For this review, use the dimensioned drawing (mm, ordinates from the lowest corner) and the shaded views. A direction names the side the tool comes from. Give positions to 0.01 mm unless a question says otherwise; leave off trailing zeros. Order: outer loops, then holes, each group sorted by start corner. A loop starts at its lowest first (then second) coordinate and runs counter-clockwise, first axis right, second up. Notation, with made-up numbers: (38, -10.5) -> (62, -10.5) arc R31 ccw to (62, 28.5) -> close; hole circle Ø3 at (81, -11.75). An arc over 180 degrees is marked (long way). One line per item, written item: value. Start each with the question number.
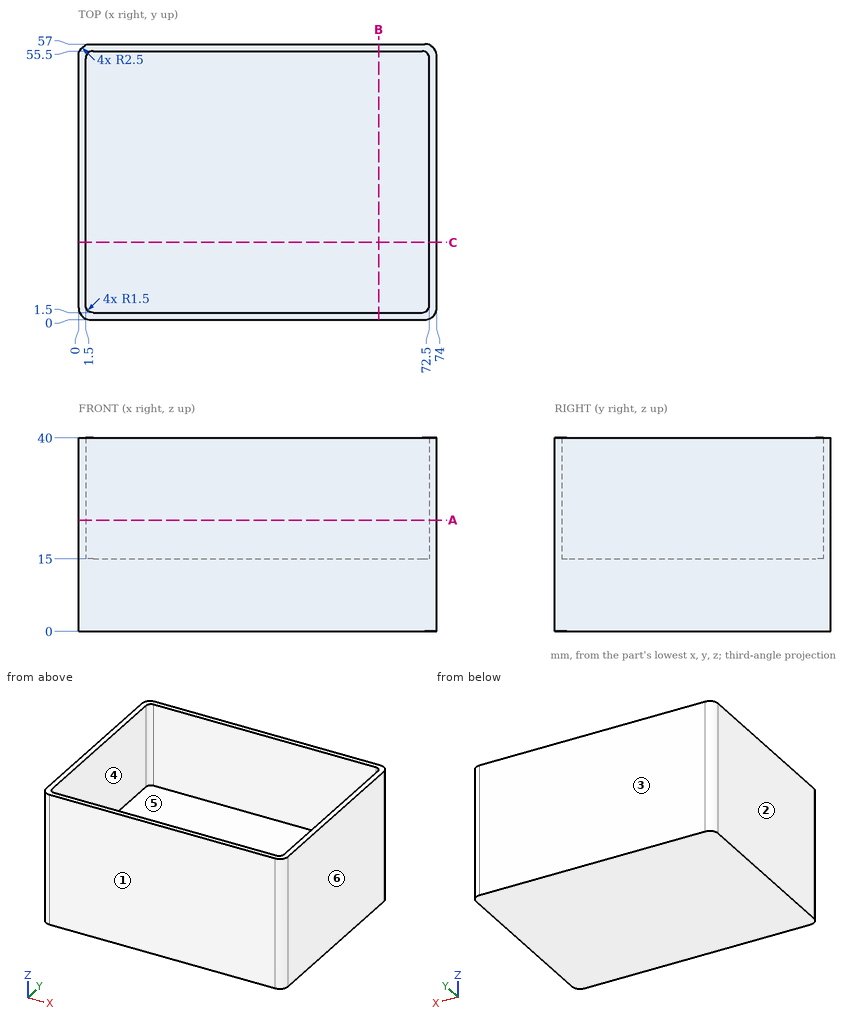
Q1. Take a section at C-C (y = 16). State the section outline as (x, z) points.
Q2. For pin 1 Ø10 at (x, y) = (33.5, 39.5) entering from +Z; pin 2 Ø6 at (x, z) = (56.5, 10) entering from -Y, all flat-tipped, find the tip position at first contact; note any pin that passes through.
Q3. For line 1 along Y through (x, z) = (28, 22); line 2 along X through (y, z) = (28, 29); line 3 along Z through (x, y) = (23, 6), list the stretches that pass through material, from the lowest coordinate up.
Q4. For the marked faces 5 and 6, list the 3-axis set-ups (+Z, -Z, +X, -X, +Y, -Y) from which the entire face can be reached by the end or side of a thin tool; tool diameter is ignored.
Q5. Take a section at B-B (x = 62). State the section outline as (y, z) points, and give its area (3 significant figures).
Q6. Take a section at A-A (z = 23). State the section outline as (x, y) points, and give its area (3 significant figures).
Q7. Mouldability with a two-part tool opening along Y and no side actions: class the marked faces 1, 2, 3 and 4 as pulls with the +Y half, pulls with the -Y half, needs draft (parallel to the pull), parting line crosses it, or undercut.
Answers below:
1. outline: (0, 0) -> (74, 0) -> (74, 40) -> (72.5, 40) -> (72.5, 15) -> (1.5, 15) -> (1.5, 40) -> (0, 40) -> close
2. pin 1: stops at z = 15
2. pin 2: stops at y = 0
3. line 1: y = 0 to 1.5, 55.5 to 57
3. line 2: x = 0 to 1.5, 72.5 to 74
3. line 3: z = 0 to 15
4. face 5: +Z
4. face 6: +Z, -Z, +X, +Y, -Y
5. outline: (0, 0) -> (57, 0) -> (57, 40) -> (55.5, 40) -> (55.5, 15) -> (1.5, 15) -> (1.5, 40) -> (0, 40) -> close
5. area: 930 mm²
6. outline: (0, 2.5) arc R2.5 ccw to (2.5, 0) -> (71.5, 0) arc R2.5 ccw to (74, 2.5) -> (74, 54.5) arc R2.5 ccw to (71.5, 57) -> (2.5, 57) arc R2.5 ccw to (0, 54.5) -> close; hole (1.5, 3) arc R1.5 ccw to (3, 1.5) -> (71, 1.5) arc R1.5 ccw to (72.5, 3) -> (72.5, 54) arc R1.5 ccw to (71, 55.5) -> (3, 55.5) arc R1.5 ccw to (1.5, 54) -> close
6. area: 381 mm²
7. face 1: pulls with the -Y half
7. face 2: needs draft
7. face 3: pulls with the +Y half
7. face 4: undercut
